The model under review builds one solid part; all positions refer to its coordinate system, in mm. A direction names the side the tool comes from. Give positions to 0.01 mm unless a question says otherwise; leave off trailing zeros. Loops run counter-clockwise (first coordinate to the right, second up) from the corner with the lowest first, then second, coordinate; pieces in that order, holes last. Notation, with made-up numbers: (41.25, -28.5) -> (83.25, -28.5) arc R17 ccw to (83.25, -11.5) -> close; hole circle Ø11 at (72, 33). An arc over 180 degrees is marked (long way). Write each question's results on one line, items separated by ' | '. Start each with the question number.
Q1. Machinability: for faces 1 (the face through (0.5, -2, 4)), 2 (the face through (4.4, -5, 3)), 3 (the face through (-2.33, -1.08, 4.87)), which of the approach directions +Z, -Z, +X, -X, +Y, -Y give a long, thin tool a straight path to every point of the face, cutting with its end or side? Answer none if there is none.
Q2. We need section A-A (z = 0). Write out the cut boundary in (x, y) (3 decimals).
Q3. We need section D-D (x = 3.75). Write out the cut boundary in (y, z) (3 decimals).
Q4. Wall thickness on L1, parallel to Z at x = -1.4, y = 0 (3 decimals); L2, parallel to Y at x = 0, z = -3.5; L3, parallel to Z at x = 4, y = -4.5: over which ranges is each line inside the solid? List them lowest first. Write a range as [from, to].
Q5. Insertion check: pin 1 Ø2 at (x, z) = (1.5, 3.5) entering from +Y; pin 2 Ø5 at (x, z) = (3.5, 3.5) entering from +Y; pin 3 Ø2 at (x, z) = (2.5, -5.5) entering from -Y. Each pin has a flat end and moves straight along its axis. Give the tip position at first contact, or say it passes through.
Q6. Mouldability with a two-part tool opening along Z and no side actions: class faces 4 (the face through (-0.04, -1.651, 7.434)), 5 (the face through (-0.5, -2, 4)), 6 (the face through (-4.4, -5, 3)) as released by +Z, released by -Z, zero draft, split by the parting line, or undercut.
Q7. We need section C-C (x = 0.75). Write out the cut boundary in (y, z) (3 decimals).
Autodesk Inventor part; units mm, degrees
ref_plane "YZ Plane" through (0, 0, 0) normal (1, 0, 0) x (0, 1, 0)
ref_plane "XZ Plane" through (0, 0, 0) normal (0, 1, 0) x (-1, 0, 0)
ref_plane "XY Plane" through (0, 0, 0) normal (0, 0, 1) x (1, 0, 0)
sketch "Sketch1" plane through (0, 0, 0) normal (0, 0, 1) x (1, 0, 0)
  line L0 (0, 0) -> (5, 0)
  line L1 (0, 0) -> (0, 20) construction
  line L2 (0, 0) -> (20, 0) construction
  line L3 (0, 4.32) -> (0.5, 4.32)
  line L4 (0.5, 4.32) -> (0.5, 4.987)
  line L5 (0.5, 4.987) -> (4.1, 4.987)
  line L6 (4.4, 5.287) -> (4.4, 6.105)
  line L7 (4.4, 6.105) -> (2.89, 7.615)
  line L8 (2.89, 7.615) -> (0, 7.615)
  line L9 (4.1, 4.987) -> (4.4, 5.287)
  line L10 (0, 4.32) -> (-0.5, 4.32)
  line L11 (-0.5, 4.32) -> (-0.5, 4.987)
  line L12 (-0.5, 4.987) -> (-4.1, 4.987)
  line L13 (-4.4, 5.287) -> (-4.4, 6.105)
  line L14 (-4.4, 6.105) -> (-2.89, 7.615)
  line L15 (-2.89, 7.615) -> (0, 7.615)
  line L16 (-4.1, 4.987) -> (-4.4, 5.287)
  point P0 (4.4, 4.987)
  point P1 (-4.4, 4.987)
  dimension "d0" = 5
  dimension "d1" = 20
  dimension "d2" = 90
  dimension "d3" = 8.64
  dimension "d4" = 15.23
  dimension "d5" = 0.5
  dimension "d6" = 3.9
  dimension "d7" = 12.21
  dimension "d8" = 9.974
  dimension "d9" = 135
  dimension "d10" = 0.3
  dimension "d11" = 0.3
  dimension "d12" = 5.78
revolve "Revolution1" add sketch "Sketch1" angle 360 about axis through (0, 0, 0) along (1, 0, 0)
properties part number "Micro V Wheel" material "Acetal Resin, Black"
Output:
1) face 1: +X | face 2: +Z, -Z, +X, +Y, -Y | face 3: -X
2) outline: (-4.4, -6.105) -> (-2.89, -7.615) -> (2.89, -7.615) -> (4.4, -6.105) -> (4.4, -5.287) -> (4.1, -4.987) -> (0.5, -4.987) -> (0.5, -4.32) -> (-0.5, -4.32) -> (-0.5, -4.987) -> (-4.1, -4.987) -> (-4.4, -5.287) -> close; (-4.4, 5.287) -> (-4.1, 4.987) -> (-0.5, 4.987) -> (-0.5, 4.32) -> (0.5, 4.32) -> (0.5, 4.987) -> (4.1, 4.987) -> (4.4, 5.287) -> (4.4, 6.105) -> (2.89, 7.615) -> (-2.89, 7.615) -> (-4.4, 6.105) -> close
3) outline: circle Ø13.51 at (0, 0); hole circle Ø9.974 at (0, 0)
4) L1: [-7.615, -4.987], [4.987, 7.615] | L2: [-6.76, -2.53], [2.53, 6.76] | L3: [-4.7, -2.15], [2.15, 4.7]
5) pin 1: y = 7.19 | pin 2: y = 7.54 | pin 3: y = -6.14
6) face 4: split by the parting line | face 5: undercut | face 6: zero draft
7) outline: circle Ø15.23 at (0, 0); hole circle Ø9.974 at (0, 0)
